```python
from build123d import *

# Parameters (mm, degrees)
ESQUISSE1_W                                 = 15.5
ESQUISSE1_H                                 = 8.312963114
ESQUISSE1_W_2                               = 10.5
ESQUISSE1_H_2                               = 12.1
ESQUISSE1_W_3                               = 12
ESQUISSE1_H_3                               = 6
BOSS_EXTRU_1_DEPTH                          = 4
FRAISAGE_POUR_VIS_T_TE_FRAIS_E_M41_AT_COUNT = 2
FRAISAGE_POUR_VIS_T_TE_FRAIS_E_M41_AT_PITCH = 22.54
FRAISAGE_POUR_VIS_T_TE_FRAIS_E_M41_2_COUNT  = 2
FRAISAGE_POUR_VIS_T_TE_FRAIS_E_M41_2_PITCH  = 75.445686424
FRAISAGE_POUR_VIS_T_TE_FRAIS_E_M41_3_COUNT  = 2
FRAISAGE_POUR_VIS_T_TE_FRAIS_E_M41_3_PITCH  = 72
CONG_1_R                                    = 1


with BuildPart() as part:
    # Esquisse1 → Boss.-Extru.1 (new body)
    with BuildSketch(Plane.XY):
        Polygon((-35.056497175, 38.54), (-35.056497175, 2), (-33.056497175, 0), (45.943502825, 0), (47.943502825, 2), (47.943502825, 38.54), (45.943502825, 40.54), (-33.056497175, 40.54), align=None)
        with Locations((-16.906497175, 13.156481557)):
            Rectangle(ESQUISSE1_W, ESQUISSE1_H, mode=Mode.SUBTRACT)
        with Locations((0.693502825, 16.05)):
            Rectangle(ESQUISSE1_W_2, ESQUISSE1_H_2, mode=Mode.SUBTRACT)
        with Locations((17.086336796, 13)):
            Rectangle(ESQUISSE1_W_3, ESQUISSE1_H_3, mode=Mode.SUBTRACT)
    extrude(amount=BOSS_EXTRU_1_DEPTH)

    # Esquisse4 → Fraisage pour vis à tête fraisée M41 (revolve, cut)
    with BuildSketch(Plane(origin=(-29.556497175, 35.54, 4), x_dir=(0, -1, 0), z_dir=(1, 0, 0))):
        Polygon((0, 0), (0, 4), (2.275, 4), (2.25, 3.975), (2.25, 2.45), (4.7, 0), align=None)
    fraisage_pour_vis_t_te_frais_e_m41 = revolve(axis=Axis((-29.556497175, 35.54, 10.35), (0, 0, -1)), mode=Mode.SUBTRACT)

    # Fraisage pour vis à tête fraisée M41 at: Fraisage pour vis à tête fraisée M41 ×2
    with Locations(*[(0, -i * FRAISAGE_POUR_VIS_T_TE_FRAIS_E_M41_AT_PITCH, 0) for i in range(1, FRAISAGE_POUR_VIS_T_TE_FRAIS_E_M41_AT_COUNT)]):
        add(fraisage_pour_vis_t_te_frais_e_m41, mode=Mode.SUBTRACT)

    # Fraisage pour vis _ t_te frais_e M41 2: Fraisage pour vis à tête fraisée M41 ×2
    with Locations(*[Vector(0.9543289141183242, -0.29875796839204205, 0) * (i * FRAISAGE_POUR_VIS_T_TE_FRAIS_E_M41_2_PITCH) for i in range(1, FRAISAGE_POUR_VIS_T_TE_FRAIS_E_M41_2_COUNT)]):
        add(fraisage_pour_vis_t_te_frais_e_m41, mode=Mode.SUBTRACT)

    # Fraisage pour vis _ t_te frais_e M41 3: Fraisage pour vis à tête fraisée M41 ×2
    with Locations(*[(i * FRAISAGE_POUR_VIS_T_TE_FRAIS_E_M41_3_PITCH, 0, 0) for i in range(1, FRAISAGE_POUR_VIS_T_TE_FRAIS_E_M41_3_COUNT)]):
        add(fraisage_pour_vis_t_te_frais_e_m41, mode=Mode.SUBTRACT)

    # Congé1
    cong_1_edges = [part.edges().sort_by_distance(p)[0] for p in [
        (-24.656497175, 17.312963114, 2),
        (-24.656497175, 9, 2),
        (-9.156497175, 9, 2),
        (-9.156497175, 17.312963114, 2),
    ]]
    fillet(cong_1_edges, radius=CONG_1_R)


solid = part.part
```
Part model, mm, in its own coordinate system. A direction names the side the tool comes from. Give positions to 0.01 mm unless a question says otherwise; leave off trailing zeros. Write each loop counter-clockwise with the first axis right and the second up, starting at its lowest first coordinate (ties: lowest second). Pieces come first, ordered by that corner, then holes. Notation, with made-up numbers: M 13,59 L 56,59 A11 ccw 56,68 Z; hole C 69.25,38 d5. An arc over 180 degrees is marked long. Use CSV: the item, a comma, the result in double quotes.
Item 1: Pull direction X, two halves, no side cores. Call faces 1 (the face through (6, 0, 2)), 2 (the face through (44.576, 34.431, 1.703)), 3 (the face through (-34.042, 39.554, 1.972)): +X half, -X half, draft (parallel to the pull), parting line (faces both ways), or undercut.
Taken from the geometry:
face 1,"draft"
face 2,"undercut"
face 3,"-X half"
Item 2: Slice it at A-A on x = -22. Write the cut outline in (y, z), plus the area to 3 significant figures.
Taken from the geometry:
outline,"M 0,0 L 9,0 L 9,4 L 0,4 Z; M 17.31,0 L 40.54,0 L 40.54,4 L 17.31,4 Z"
area,"129 mm²"
Item 3: Slice it at D-D on z = 0.7. Write the cut outline in (x, y), plus the area to 3 significant figures.
Taken from the geometry:
outline,"M -35.06,2 L -33.06,0 L 45.94,0 L 47.94,2 L 47.94,38.54 L 45.94,40.54 L -33.06,40.54 L -35.06,38.54 Z; hole C -29.56,13 d4.5; hole C -29.56,35.54 d4.5; hole M -24.66,10 A1 ccw -23.66,9 L -10.16,9 A1 ccw -9.16,10 L -9.16,16.31 A1 ccw -10.16,17.31 L -23.66,17.31 A1 ccw -24.66,16.31 Z; hole M -4.56,10 L 5.94,10 L 5.94,22.1 L -4.56,22.1 Z; hole M 11.09,10 L 23.09,10 L 23.09,16 L 11.09,16 Z; hole C 42.44,13 d4.5; hole C 42.44,35.54 d4.5"
area,"2,970 mm²"
Item 4: Drill centre lines: probe 1 along X at (y, z) = (13, 0.75); probe 2 along X at (y, z) = (21.5, 1.3); probe 3 along Y at (x, z) = (12.5, 3.3). Where is each one in solid material? Low to high.
Taken from the geometry:
probe 1,"x = -35.06 to -31.81, -27.31 to -24.66, -9.16 to -4.56, 5.94 to 11.09, 23.09 to 40.19, 44.69 to 47.94"
probe 2,"x = -35.06 to -4.56, 5.94 to 47.94"
probe 3,"y = 0 to 10, 16 to 40.54"
Item 5: Slice it at B-B on y = 35.54. State how many separate pieces and enclosed holes the cut face has, plus the area to 3 significant figures.
Taken from the geometry:
separate pieces,"3"
enclosed holes,"0"
area,"284 mm²"
Item 6: Pin check, flat tip, straight feed: P1, Ø2, axis at x = 27, z = 2, coming from the -Y side. Stop position of the tip, or through.
Taken from the geometry:
P1,"stops at y = 0"
Item 7: Which spindle directions (+Z, -Z, +X, -X, +Y, -Y) get a long thin tool onto all of the face, cutting with end or side? Do faces 4 (the face through (-34.07, 1.014, 1.972)), 5 (the face through (-24.656, 13, 2)). Say none if no direction does.
Taken from the geometry:
face 4,"+Z, -Z, -X, -Y"
face 5,"+Z, -Z"
